Autodesk Inventor part; units mm, degrees
ref_plane "Work Plane1" through (17.5, 30.3109, 22) normal (0.5, 0.866, 0) x (-0.866, 0.5, 0)
ref_plane "Work Plane2" through (26.8116, 22.4976, 22) normal (0.766, 0.6428, 0) x (-0.6428, 0.766, 0)
ref_plane "Work Plane3" through (-17.5, 30.3109, 22) normal (-0.5, 0.866, 0) x (-0.866, -0.5, 0)
sketch "Sketch1" plane through (0, 0, 0) normal (0, 0, 1) x (1, 0, 0)
  circle A0 centre (0, 0) radius 35
  circle A1 centre (0, 0) radius 12
  dimension "d0" = 70
  dimension "d1" = 24
extrude "Extrusion1" add sketch "Sketch1" along normal blind 22
sketch "Sketch2" plane through (0, 0, 22) normal (0, 0, 1) x (1, 0, 0)
  circle A0 centre (0, 0) radius 12
  circle A1 centre (0, 0) radius 35
  circle A2 centre (0, 0) radius 25.5
  circle A3 centre (0, 0) radius 19.5
  dimension "d4" = 51
  dimension "d5" = 6
extrude "Extrusion2" cut sketch "Sketch2" against normal blind 2.1 contours A2
sketch "Sketch3" plane through (0, 0, 22) normal (0, 0, 1) x (1, 0, 0)
  line L0 (0, 0) -> (0, 45.779) construction
  line L1 (0, 0) -> (38.81, 0) construction
  line L2 (0, 0) -> (26.8116, 22.4976) construction
  circle A0 centre (0, 0) radius 35 construction
  line L3 (0, 0) -> (35, 0) construction
  line L4 (0, 0) -> (17.5, 30.3109) construction
  line L5 (0, 0) -> (35, 0) construction
  line L6 (0, 0) -> (-26.8116, 22.4976) construction
  line L7 (0, 0) -> (-17.5, 30.3109) construction
  dimension "d11" = 40
  dimension "d12" = 60
ref_plane "Work Plane1" through (17.5, 30.3109, 22) normal (0.5, 0.866, 0) x (-0.866, 0.5, 0)
ref_plane "Work Plane2" through (26.8116, 22.4976, 22) normal (0.766, 0.6428, 0) x (-0.6428, 0.766, 0)
ref_plane "Work Plane3" through (-17.5, 30.3109, 22) normal (-0.5, 0.866, 0) x (-0.866, -0.5, 0)
ref_plane "Work Plane4" through (-26.8116, 22.4976, 22) normal (-0.766, 0.6428, 0) x (-0.6428, -0.766, 0)
sketch "Sketch4" plane through (26.8116, 22.4976, 22) normal (0.766, 0.6428, 0) x (-0.6428, 0.766, 0)
  line L0 (35, 0) -> (-35, 0)
  point P0 (0, -22)
  point P1 (0, -13)
  dimension "d13" = 13
hole "Hole1" at (26.8116, 22.4976, 9) direction (-0.766, -0.6428, 0) diameter 3 depth 4 tip angle 118
sketch "Sketch5" plane through (17.5, 30.3109, 22) normal (0.5, 0.866, 0) x (-0.866, 0.5, 0)
  line L0 (35, 0) -> (-35, 0)
  point P0 (0, -22)
  point P1 (0, -13)
  dimension "d21" = 13
hole "Hole2" at (17.5, 30.3109, 9) direction (-0.5, -0.866, 0) diameter 3 depth 8 tip angle 118
sketch "Sketch6" plane through (-17.5, 30.3109, 22) normal (-0.5, 0.866, 0) x (-0.866, -0.5, 0)
  line L0 (35, 0) -> (-35, 0)
  point P0 (0, -22)
  point P1 (0, -13)
  dimension "d29" = 13
hole "Hole3" at (-17.5, 30.3109, 9) direction (0.5, -0.866, 0) diameter 3 depth 8 tip angle 118
sketch "Sketch7" plane through (-26.8116, 22.4976, 22) normal (-0.766, 0.6428, 0) x (-0.6428, -0.766, 0)
  line L0 (35, 0) -> (-35, 0)
  point P0 (0, -22)
  point P1 (0, -13)
  dimension "d37" = 13
hole "Hole4" at (-26.8116, 22.4976, 9) direction (0.766, -0.6428, 0) diameter 3 depth 8 tip angle 118
thread "Thread1"
thread "Thread2"
thread "Thread3"
thread "Thread4"
sketch "Sketch9" plane through (0, 0, 22) normal (0, 0, 1) x (1, 0, 0)
  circle A0 centre (0, 0) radius 16
  dimension "d53" = 32
extrude "Extrusion3" cut sketch "Sketch9" against normal blind 18
sketch "Sketch11" plane through (0, 0, 0) normal (0, 0, -1) x (-1, 0, 0)
  circle A0 centre (0, 0) radius 27 construction
  point P0 (-27, 0)
  point P1 (0, -27)
  point P2 (27, 0)
  point P3 (0, 27)
  dimension "d77" = 54
  dimension "d80" = 360
hole "Hole6" at (27, 0, 0) at (0, -27, 0) at (-27, 0, 0) at (0, 27, 0) direction (0, 0, 1) diameter 3 depth 8 tip angle 118
thread "Thread9"
thread "Thread10"
thread "Thread11"
thread "Thread12"
chamfer "Chamfer2" distance 2 angle 45 1 edges at (-35, 0, 0)
properties part number "joint_mag_side" material "Aluminum 6061"
Verification items for the finished model (mm, model axes). A direction names the side the tool comes from. Round coordinates to 2 decimals unless told otherwise and drop trailing zeros. Loops run counter-clockwise (first coordinate to the right, second up) from the corner with the lowest first, then second, coordinate; pieces in that order, holes last. Notation, with made-up numbers: (73, 30) -> (108, 30) arc R17 cw to (108, 43) -> close; hole circle Ø1 at (10, -15). An arc over 180 degrees is marked (long way). Answer as a JSON object with one key per item and string values.
Q1. Section check A-A (z = 6.25). Record the boundary of the cut face in (x, y), then the cut area to 3 significant figures.
Data:
{"outline": "circle Ø70 at (0, 0); hole circle Ø3 at (-27, 0); hole circle Ø32 at (0, 0); hole circle Ø3 at (0, -27); hole circle Ø3 at (0, 27); hole circle Ø3 at (27, 0)", "area": "3,020 mm2"}
Q2. Access from +Z, -Z, +X, -X, +Y, -Y to the whole of each face (thin tool, end or side, straight path). Record for faces 4 (the cylindrical face through (-0.07, 25.5, 4.06)), 5 (the flat face through (2, 12, 4)), 6 (the conical face through (-13.06, 22.78, 9.25)).
Data:
{"face 4": "-Z", "face 5": "+Z", "face 6": "none"}
Q3. Go/stop test with flat-tipped pins: P1, Ø8, axis at x = 18.5, y = -14, coming from the -Z side; P2, Ø2.5, axis at x = -27, y = 0, coming from the -Z side; P3, Ø12, axis at x = -2.5, z = 15, coming from the +Y side; P4, Ø6, axis at y = 10, z = 15.5, coming from the +X side. Record where each tip stops, or that it passes through.
Data:
{"P1": "stops at z = 0", "P2": "stops at z = 8.15", "P3": "stops at y = 35", "P4": "stops at x = 34.29"}
Q4. Draft check along Y on faces 1 (the cylindrical face through (-5.5, -24.9, 21)), 2 (the cylindrical face through (-28, 21, 12)), 3 (the flat face through (3, 16, 22)). Enter one of: pulls with the +Y half, pulls with the -Y half, needs draft (parallel to the pull), parting line crosses it, or undercut.
Data:
{"face 1": "undercut", "face 2": "parting line crosses it", "face 3": "needs draft"}
Q5. Scan lines: line 1 (Y direction, x = 0, z = 13.5); line 2 (Y direction, x = 14.5, z = 21); line 3 (Y direction, x = -14, z = 9.5). Record each from-to range of solid material in increasing order. Write a range as from..to.
Data:
{"line 1": "y = -35..-16, 16..35", "line 2": "y = -31.86..-20.98, -13.04..-6.76, 6.76..13.04, 20.98..31.86", "line 3": "y = -32.08..-7.75, 7.75..22.69, 27.08..32.08"}
